Verification items for this drawing (mm, ordinates from the low corner). A direction names the side the tool comes from. Give positions to 0.01 mm unless a question says otherwise; leave off trailing zeros. Loops run counter-clockwise (first coordinate to the right, second up) from the corner with the lowest first, then second, coordinate; pieces in that order, holes last. Notation, with made-up numbers: (-4, -27) -> (12, -27) arc R20 ccw to (12, -10) -> close; hole circle Ø8 at (39, -3.75). An arc over 180 degrees is marked (long way). Answer as CSV lines item,"result". Start each with the question number.
(1) Gauge pin test, flat ends, axial feed: pin 1 Ø0.8 at (x, z) = (6.5, 49) entering from +Y; pin 2 Ø8 at (x, z) = (26, 16) entering from -Y; pin 3 Ø2 at (y, z) = (1.5, 30) entering from -X; pin 4 Ø3 at (x, z) = (18.5, 44) entering from +Y. Record the tip position at first contact, or that the pin passes through.
(2) Material ranges on line 1 (Z direction, x = 29.75, y = 7.5); line 2 (X direction, y = 7.5, z = 6); line 3 (Z direction, x = 7.25, y = 4.5), recorded low to high. Write a range as from..to.
(3) Section check C-C on z = 20. Enter the section's corners in (x, y).
(4) Release check for a two-part mould opening along Z. For the marked faces 5, 6 and 7 record: pulls with the +Z half, pulls with the -Z half, needs draft (parallel to the pull), parting line crosses it, or undercut.
(5) Access from +Z, -Z, +X, -X, +Y, -Y to the whole of each face (thin tool, end or side, straight path). Record for the marked faces 1, 2, 3 and 4.
(6) Section check A-A on y = 11.25. Enter the section's corners in (x, z), plus the area to 3 significant figures.
(7) Section check B-B on z = 6. State how many separate pieces and enclosed holes the cut face has, plus the area to 3 significant figures.
(8) Section check D-D on x = 24. Enter the section's corners in (y, z), plus the area to 3 significant figures.
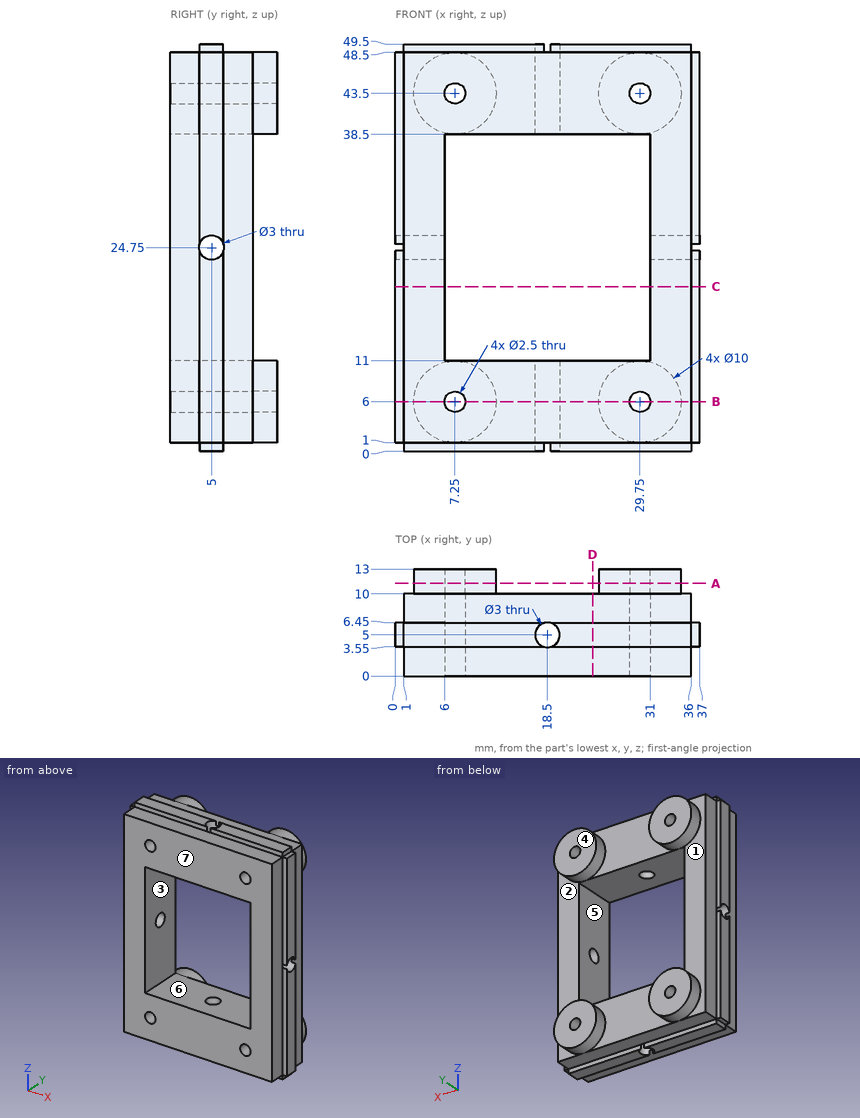
Working result:
1,pin 1,"stops at y = 6.45"
1,pin 2,"passes through"
1,pin 3,"stops at x = 1"
1,pin 4,"stops at y = 10"
2,line 1,"z = 1..4.75, 7.25..11, 38.5..42.25, 44.75..48.5"
2,line 2,"x = 1..6, 8.5..28.5, 31..36"
2,line 3,"z = 0..4.75, 7.25..11, 38.5..42.25, 44.75..49.5"
3,outline,"(0, 3.55) -> (1, 3.55) -> (1, 0) -> (6, 0) -> (6, 10) -> (1, 10) -> (1, 6.45) -> (0, 6.45) -> close; (31, 0) -> (36, 0) -> (36, 3.55) -> (37, 3.55) -> (37, 6.45) -> (36, 6.45) -> (36, 10) -> (31, 10) -> close"
4,face 5,"undercut"
4,face 6,"undercut"
4,face 7,"needs draft"
5,face 1,"-X, +Y"
5,face 2,"+X, +Y"
5,face 3,"+Y, -Y"
5,face 4,"+Z, -Z, +X, -X, +Y"
6,outline,"circle Ø10 at (7.25, 6); circle Ø10 at (7.25, 43.5); circle Ø10 at (29.75, 6); circle Ø10 at (29.75, 43.5); hole circle Ø2.5 at (7.25, 6); hole circle Ø2.5 at (7.25, 43.5); hole circle Ø2.5 at (29.75, 6); hole circle Ø2.5 at (29.75, 43.5)"
6,area,"295 mm^2"
7,separate pieces,"3"
7,enclosed holes,"1"
7,area,"344 mm^2"
8,outline,"(0, 1) -> (3.55, 1) -> (3.55, 0) -> (6.45, 0) -> (6.45, 1) -> (10, 1) -> (10, 11) -> (0, 11) -> close; (0, 38.5) -> (10, 38.5) -> (10, 48.5) -> (6.45, 48.5) -> (6.45, 49.5) -> (3.55, 49.5) -> (3.55, 48.5) -> (0, 48.5) -> close"
8,area,"206 mm^2"
